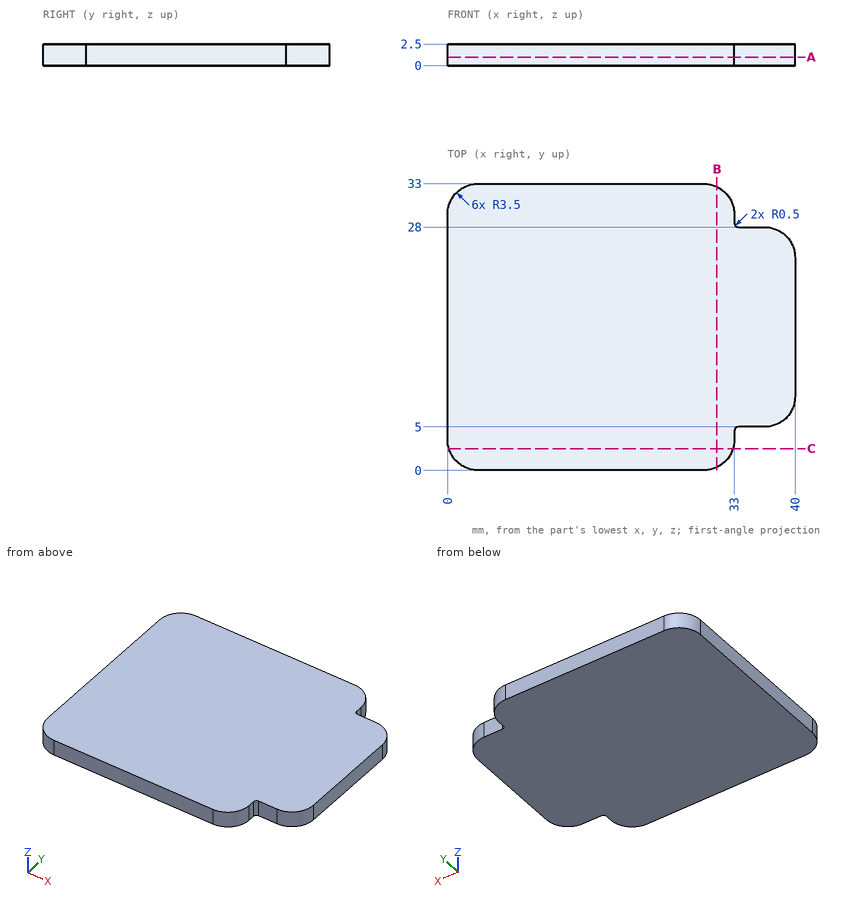
Source: three-view drawing plus pictorial views. Frame: mm from the lowest corner of the part. Coordinates: 2 decimals unless noted, no trailing zeros. Loops run counter-clockwise (first coordinate to the right, second up) from the corner with the lowest first, then second, coordinate; pieces in that order, holes last. Notation, with made-up numbers: (70, 13.25) - (119, 13.25) arc R31 ccw to (119, 52.25) - close; hole circle Ø3 at (73, 52.5). An arc over 180 degrees is marked (long way). One line per item, written item: value. Start each with the question number.
1. Section B-B (x = 31). Return the cut outline in (y, z).
2. Ray query, L1, parallel to Y at x = 36.5, z = 0.25; L2, parallel to X at y = 4, z = 0.5; L3, parallel to Y at x = 32, z = 2.2. Return the intervals inside material, ascending.
3. Section A-A (z = 1). Return the cut outline in (x, y).
4. Contact query for flat-ended pins moving along their axis: P1, Ø10, axis at x = 22, y = 14.5, coming from the -Z side; P2, Ø1.1, axis at y = 29, z = 1, coming from the +X side. Output: stop coordinate, or through.
5. Section C-C (y = 2.5). Return the cut outline in (x, z), and give its area (3 significant figures).
Verdict:
1. outline: (0.34, 0) - (32.66, 0) - (32.66, 2.5) - (0.34, 2.5) - close
2. L1: y = 5 to 28
2. L2: x = 0 to 33
2. L3: y = 1.05 to 31.95
3. outline: (0, 3.5) arc R3.5 ccw to (3.5, 0) - (29.5, 0) arc R3.5 ccw to (33, 3.5) - (33, 4.5) arc R0.5 cw to (33.5, 5) - (36.5, 5) arc R3.5 ccw to (40, 8.5) - (40, 24.5) arc R3.5 ccw to (36.5, 28) - (33.5, 28) arc R0.5 cw to (33, 28.5) - (33, 29.5) arc R3.5 ccw to (29.5, 33) - (3.5, 33) arc R3.5 ccw to (0, 29.5) - close
4. P1: stops at z = 0
4. P2: stops at x = 33
5. outline: (0.15, 0) - (32.85, 0) - (32.85, 2.5) - (0.15, 2.5) - close
5. area: 81.8 mm2
